Geometry: see drawing. Coordinates: mm, zero at the bounding-box minimum. Coordinates: 2 decimals unless noted, no trailing zeros. Loops run counter-clockwise (first coordinate to the right, second up) from the corner with the lowest first, then second, coordinate; pieces in that order, holes last. Notation, with made-up numbers: M 41,72.5 L 82,72.5 A18 cw 82,97.5 Z; hole C 58.25,30.5 d4. An arc over 180 degrees is marked long. One line per question, with ' | ' between items. Start each with the question number.
1. Section query A-A, the plane y = 10.25. Output: boundary loops of the cut face in (x, z), and give its area (3 significant figures).
2. Section query B-B, the plane z = 77. Output: boundary loops of the cut face in (x, y).
3. Section query D-D, the plane x = 28. Output: boundary loops of the cut face in (y, z).
4. Ray query, probe 1 along X at (y, z) = (10, 135); probe 2 along Y at (x, z) = (54, 129). Return the intervals inside material, ascending.
5. Pin query (flat end, axial travel): P1, Ø8, axis at y = 2.5, z = 122, coming from the +X side; P2, Ø2, axis at x = 124, y = 6.5, coming from the +Z side; P3, Ø1.2, axis at x = 95.5, y = 2.5, coming from the +Z side. Return the tip coordinate at first contact, or that it passes through.
6. Mould query, pull axis X, two halves, no side actions, for the marked faces 1, 2 and 3. Classes: pulls with the +X half, pulls with the -X half, needs draft (parallel to the pull), parting line crosses it, or undercut.
7. Section query C-C, the plane x = 60.5. Output: boundary loops of the cut face in (y, z) (1 decimal).
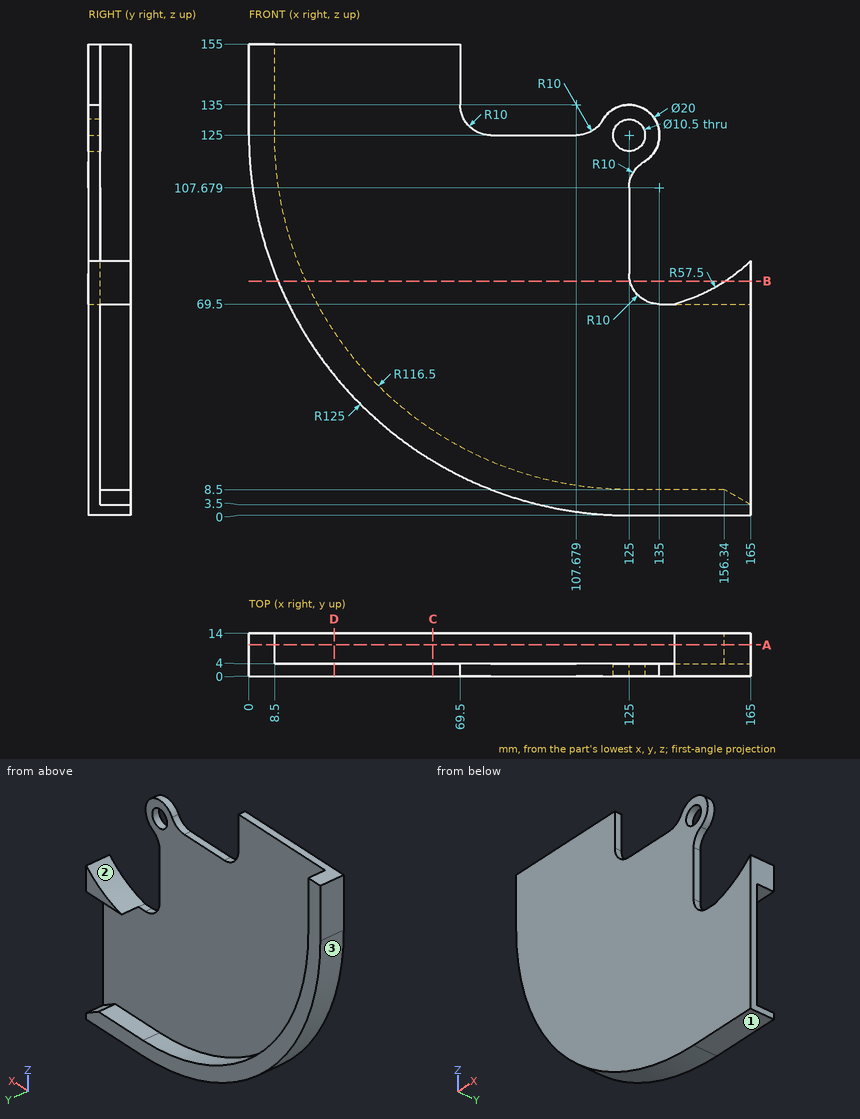
Taken from the geometry:
1) outline: M 0,125 A125 ccw 125,0 L 165,0 L 165,3.5 L 156.34,8.5 L 125,8.5 A116.5 cw 8.5,125 L 8.5,155 L 0,155 Z; M 140.03,69.5 L 165,69.5 L 165,83.69 A57.5 cw Z | area: 2,330 mm^2
2) outline: M 9.58,0 L 125.32,0 L 125.32,4 L 18.85,4 L 18.85,14 L 9.58,14 Z; M 156.66,0 L 165,0 L 165,14 L 156.66,14 Z
3) outline: M 0,46.16 L 14,46.16 L 14,60.48 L 4,60.48 L 4,155 L 0,155 Z
4) probe 1: 0 to 8.5 | probe 2: 0 to 4
5) P1: x = 135 | P2: z = 8.52 | P3: z = 125
6) face 1: needs draft | face 2: undercut | face 3: pulls with the -X half
7) outline: M 0,17.9 L 14,17.9 L 14,28 L 4,28 L 4,155 L 0,155 Z
